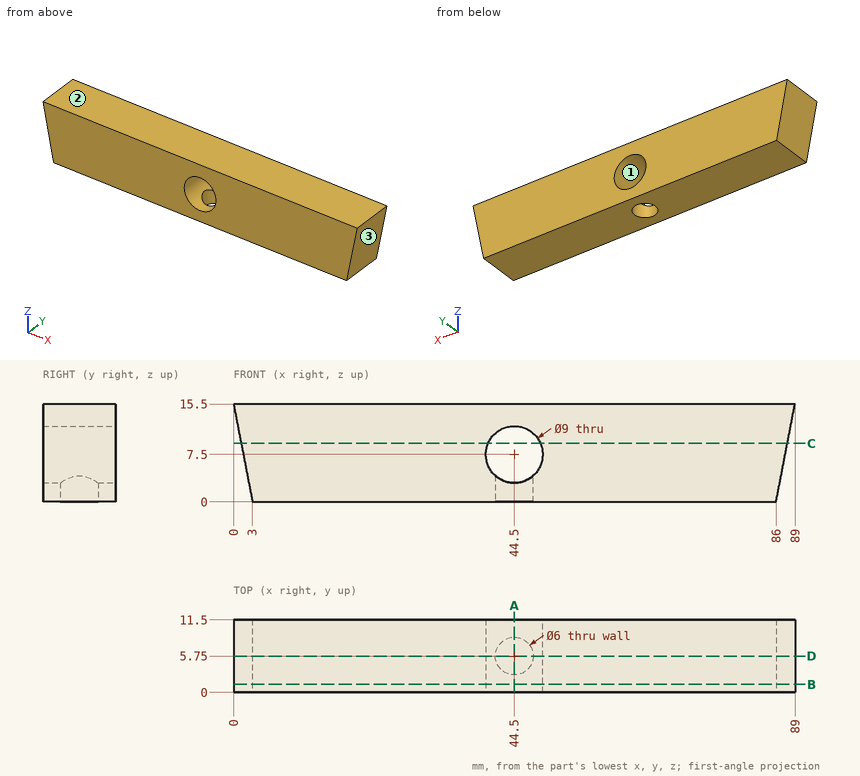
The figure shows three views and two pictorial views of one solid part (mm, origin at its lowest corner). Answer the questions. Coordinates: 2 decimals unless noted, no trailing zeros. Loops run counter-clockwise (first coordinate to the right, second up) from the corner with the lowest first, then second, coordinate; pieces in that order, holes last. Notation, with made-up numbers: (27, 38) - (47, 38) arc R22 cw to (47, 58) - close; hole circle Ø9 at (63, 18.25). An arc over 180 degrees is marked (long way). Write item = value, one per line.
1) Section B-B (y = 1.25) is taken. Determine the outline of the cut face in (x, z), plus the area to 3 significant figures.
Responses:
outline = (0, 15.5) - (3, 0) - (86, 0) - (89, 15.5) - close; hole circle Ø9 at (44.5, 7.5)
area = 1,270 mm^2
2) Determine the mould class of the marked faces 1, 2 and 3 for opening direction Z: pulls with the +Z half, pulls with the -Z half, needs draft (parallel to the pull), parting line crosses it, or undercut.
Responses:
face_1 = undercut
face_2 = pulls with the +Z half
face_3 = pulls with the -Z half
3) Section A-A (x = 44.5) is taken. Determine the outline of the cut face in (y, z), plus the area to 4 significant figures.
Responses:
outline = (0, 0) - (2.75, 0) - (2.75, 3) - (0, 3) - close; (0, 12) - (11.5, 12) - (11.5, 15.5) - (0, 15.5) - close; (8.75, 0) - (11.5, 0) - (11.5, 3) - (8.75, 3) - close
area = 56.75 mm^2
4) Section D-D (y = 5.75) is taken. Determine the outline of the cut face in (x, z), plus the area to 3 significant figures.
Responses:
outline = (0, 15.5) - (3, 0) - (41.5, 0) - (41.5, 4.15) arc R4.5 cw (long way) to (47.5, 4.15) - (47.5, 0) - (86, 0) - (89, 15.5) - close
area = 1,250 mm^2
5) Section C-C (z = 9.25) is taken. Determine the outline of the cut face in (x, y), plus the area to 3 significant figures.
Responses:
outline = (1.21, 0) - (40.35, 0) - (40.35, 11.5) - (1.21, 11.5) - close; (48.65, 0) - (87.79, 0) - (87.79, 11.5) - (48.65, 11.5) - close
area = 900 mm^2
6) This flat-tipped pin is pushed along its axis until it touches: P1, Ø5, axis at x = 44.5, y = 5.75, coming from the -Z side. Where does it stop, or does it pass through?
Responses:
P1 = 11.24
7) Find the intervals of material crossed by line 1 along X through (y, z) = (7.5, 6.5); line 2 along Z through (x, y) = (44.5, 4.5); line 3 along Y through (x, z) = (44.5, 1.15), in increasing order.
Responses:
line_1 = 1.74 to 40.11, 48.89 to 87.26
line_2 = 12 to 15.5
line_3 = 0 to 2.75, 8.75 to 11.5
